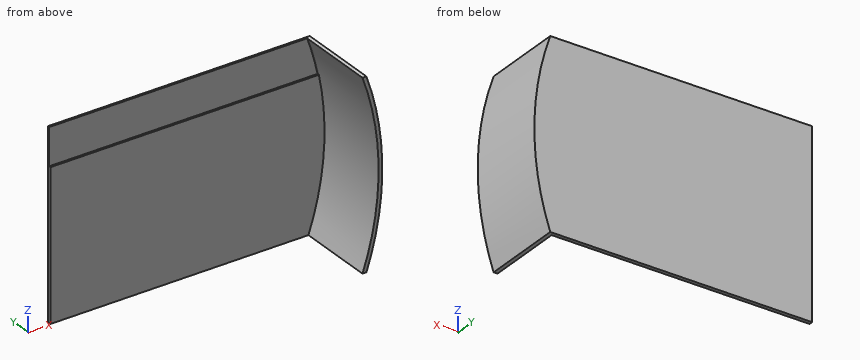
```python
from build123d import *

# Parameters (mm, degrees)
BOSS_EXTRUDE1_DEPTH = 44
SHELL1_T            = -2
CUT_EXTRUDE1_DEPTH  = 1


with BuildPart() as part:
    # Sketch1 → Boss-Extrude1 (new body)
    with BuildSketch(Plane(origin=(0, 0, 0), x_dir=(1, 0, 0), z_dir=(0, 1, 0))):
        with BuildLine():
            Line((0, 0), (0, 50))
            Line((0, 50), (141.421356237, 50))
            ThreePointArc((141.421356237, 50), (150, 0), (141.421356237, -50))
            Line((141.421356237, -50), (0, -50))
            Line((0, -50), (0, 0))
        make_face()
    extrude(amount=BOSS_EXTRUDE1_DEPTH)

    # Shell1
    shell1_openings = [part.faces().sort_by_distance(p)[0] for p in [
        (70.710678119, 22, 50),
        (73.609024715, 0, 0),
        (0, 22, 0),
        (70.710678119, 22, -50),
    ]]
    offset(amount=SHELL1_T, openings=shell1_openings, kind=Kind.INTERSECTION)

    # Sketch3 → Cut-Extrude1 (cut)
    with BuildSketch(Plane.XZ.offset(-42)):
        with BuildLine():
            Line((0, 30), (144.927568116, 30))
            ThreePointArc((144.927568116, 30), (142.464303142, 40.098906848), (139.298241195, 50))
            Line((139.298241195, 50), (0, 50))
            Line((0, 50), (0, 30))
        make_face()
    extrude(amount=-CUT_EXTRUDE1_DEPTH, mode=Mode.SUBTRACT)


solid = part.part
```
Here's how the part is built. I have some questions about the finished solid (model axes, mm). Round coordinates to 2 decimals unless told otherwise and drop trailing zeros. Loops run counter-clockwise (first coordinate to the right, second up) from the corner with the lowest first, then second, coordinate; pieces in that order, holes last.
1. Will these pins go through, and if not, where does the flat tip stop? pin 1 (10 mm diameter, centred on x = 70, y = 36, fed in from -Z); pin 2 (4 mm diameter, centred on x = 65.5, z = -9, fed in from -Y); pin 3 (6 mm diameter, centred on x = 44.5, z = 37.5, fed in from -Y); pin 4 (1 mm diameter, centred on y = 38.5, z = -28.5, fed in from -X).
Answers:
pin 1: passes through
pin 2: stops at y = 42
pin 3: stops at y = 43
pin 4: stops at x = 145.13
2. If I drill on probe 1 along Y at (x, z) = (27, -16.5); probe 2 along Y at (x, z) = (38, 37); probe 3 along X at (y, z) = (11, 42.5), over which ranges is the centre line in solid material (lowest first)?
Answers:
probe 1: y = 42 to 44
probe 2: y = 43 to 44
probe 3: x = 141.77 to 143.85
3. Suppose I cut it at A-A, the plane x = 137.5. Please give me the cut outline in (y, z).
Answers:
outline: (42, -50) - (44, -50) - (44, 50) - (43, 50) - (43, 30) - (42, 30) - close
4. Suppose I cut it at C-C, the plane z = 33.5. Please give me the cut outline in (x, y), and give its area (3 significant figures).
Answers:
outline: (0, 43) - (144.16, 43) - (144.16, 0) - (146.21, 0) - (146.21, 44) - (0, 44) - close
area: 234 mm2
5. Suppose I cut it at D-D, the plane z = -1. Please give me the cut outline in (x, y), and give its area (3 significant figures).
Answers:
outline: (0, 42) - (148, 42) - (148, 0) - (150, 0) - (150, 44) - (0, 44) - close
area: 384 mm2
6. Suppose I cut it at B-B, the plane y = 26. Please give me the cut outline in (x, z), and give its area (3 significant figures).
Answers:
outline: (139.3, -50) - (141.42, -50) arc R150 ccw to (141.42, 50) - (139.3, 50) arc R148 cw to start
area: 204 mm2
